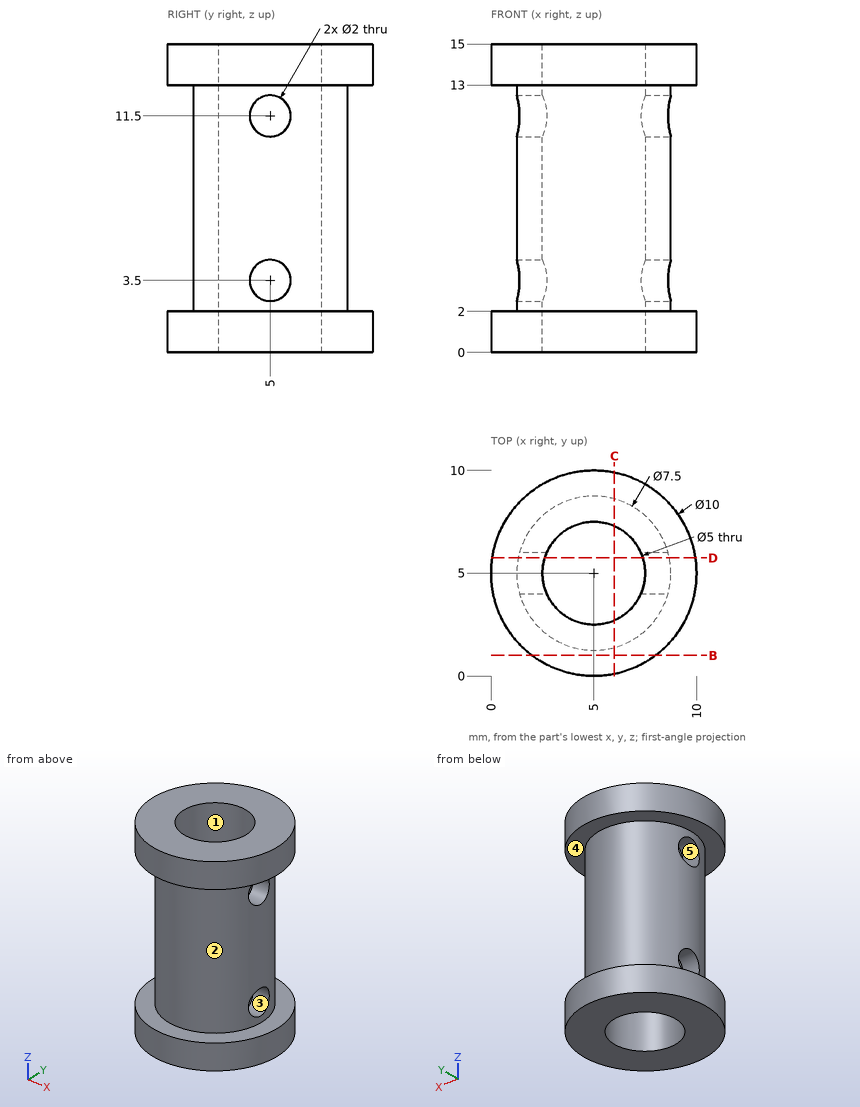
Source: three-view drawing plus pictorial views. Frame: mm from the lowest corner of the part. A direction names the side the tool comes from. Give positions to 0.01 mm unless a question says otherwise; leave off trailing zeros. Write each loop counter-clockwise with the first axis right and the second up, starting at its lowest first coordinate (ties: lowest second). Pieces come first, ordered by that corner, then holes. Notation, with made-up numbers: M 41,-34.5 L 76,-34.5 A3 cw 76,-30.5 Z; hole C 26,-3 d9. An arc over 180 degrees is marked long. Use one line per item in the form item = value.
1. Reachability of the marked faces 4 and 5 from +Z, -Z, +X, -X, +Y, -Y: full face, straight path, thin tool, end or side. Return the list, or none.
Outcome:
face_4 = none
face_5 = +X, -X
2. Cut plane C-C on x = 6. Return loops of the section in (y, z) (1 decimal).
Outcome:
outline = M 0.1,0 L 2.7,0 L 2.7,15 L 0.1,15 L 0.1,13 L 1.4,13 L 1.4,2 L 0.1,2 Z; M 7.3,0 L 9.9,0 L 9.9,2 L 8.6,2 L 8.6,13 L 9.9,13 L 9.9,15 L 7.3,15 Z
3. Mould query, pull axis X, two halves, no side actions, for the marked faces 1, 2 and 3. Classes: released by +X, released by -X, zero draft, split by the parting line, or undercut.
Outcome:
face_1 = undercut
face_2 = split by the parting line
face_3 = zero draft
4. Ray query, L1, parallel to Z at x = 1, y = 3.5; L2, parallel to X at y = 5.5, z = 9.75; L3, parallel to Y at x = 6, z = 14. Return the intervals inside material, ascending.
Outcome:
L1 = 0 to 2, 13 to 15
L2 = 1.28 to 2.55, 7.45 to 8.72
L3 = 0.1 to 2.71, 7.29 to 9.9
5. Cut plane D-D on y = 5.75. State how many separate pieces and enclosed holes the cut face has.
Outcome:
separate_pieces = 6
enclosed_holes = 0
6. Cut plane B-B on y = 1. Return loops of the section in (x, z), and give its area (3 significant figures).
Outcome:
outline = M 2,0 L 8,0 L 8,2 L 2,2 Z; M 2,13 L 8,13 L 8,15 L 2,15 Z
area = 24.0 mm²
7. First-contact query: P1, Ø1.5, axis at x = 2.5, z = 7.5, coming from the -Y side; P2, Ø2.5, axis at y = 5, z = 11.5, coming from the -X side; P3, Ø1.5, axis at y = 8.5, z = 11, coming from the +X side. Flat tips, straight axial feed; report the tip coordinate or a pass-through.
Outcome:
P1 = 1.68
P2 = 1.25
P3 = 7.55
